Autodesk Inventor part; units mm, degrees
ref_plane "YZ Plane" through (0, 0, 0) normal (1, 0, 0) x (0, 1, 0)
ref_plane "XZ Plane" through (0, 0, 0) normal (0, 1, 0) x (-1, 0, 0)
ref_plane "XY Plane" through (0, 0, 0) normal (0, 0, 1) x (1, 0, 0)
sketch "Boceto2" plane through (0, 0, 0) normal (0, 1, 0) x (-1, 0, 0)
  line L0 (0, 0) -> (-78, 0)
  line L1 (-78, 0) -> (-78, -30)
  line L2 (-78, -30) -> (-38, -30)
  line L3 (-38, -30) -> (-38, -36)
  line L4 (-38, -36) -> (0, -36)
  line L5 (0, -36) -> (0, 0)
  dimension "d2" = 78
  dimension "d3" = 36
  dimension "d4" = 30
  dimension "d5" = 38
extrude "Extrusión1" add sketch "Boceto2" along normal blind 38
sketch "Boceto3" plane through (0, 0, -36) normal (-1, 0, 0) x (0, 0, 1)
  line L0 (0, 0) -> (36, 0) construction
  line L1 (36, 0) -> (36, 6) construction
  line L2 (36, 0) -> (36, 38) construction
  line L3 (36, 6) -> (36, 27) construction
  line L4 (36, 27) -> (36, 38) construction
  line L5 (36, 6) -> (18, 6)
  line L6 (18, 6) -> (18, 27)
  line L7 (18, 27) -> (36, 27)
  line L8 (36, 6) -> (36, 27)
  dimension "d8" = 6
  dimension "d9" = 21
  dimension "d10" = 38
  dimension "d11" = 18
extrude "Extrusión2" cut sketch "Boceto3" against normal through all
sketch "Boceto4" plane through (38, 0, -36) normal (0, 0, -1) x (-1, 0, 0)
  line L0 (38, 27) -> (38, 38) construction
  line L1 (38, 38) -> (38, 19) construction
  line L2 (38, 19) -> (19, 19) construction
  line L3 (0, 0) -> (0, 38) construction
  circle A0 centre (19, 19) radius 8
  point P0 (38, 0)
  dimension "d14" = 19
  dimension "d15" = 19
  dimension "d16" = 16
extrude "Extrusión3" cut sketch "Boceto4" against normal through all
chamfer "Chaflán1" distance 2 angle 45 4 edges at (19, 38, -36) (0, 19, -36) (19, 0, -36) (38, 19, -36)
properties part number "Practica 6"
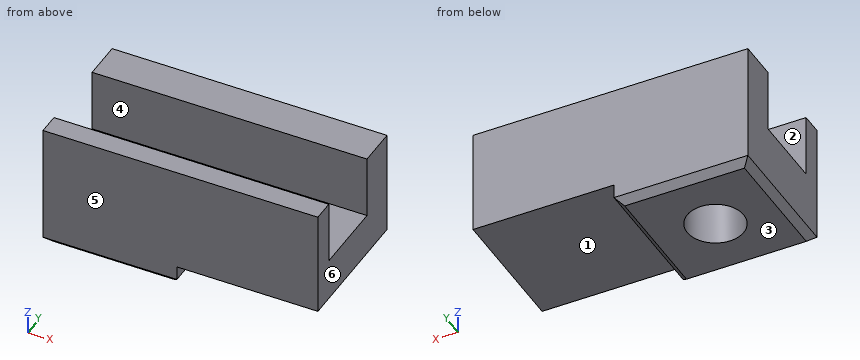
Geometry: final body of the model. Coordinates: model frame, mm. Face numbers are marked on the shaded views. A direction names the side the tool comes from. Give positions to 0.01 mm unless a question says otherwise; leave off trailing zeros. Write each loop counter-clockwise with the first axis right and the second up, starting at its lowest first coordinate (ties: lowest second). Pieces come first, ordered by that corner, then holes.
(1) Cut plane C-C, the plane x = 16.5. Return loops of the section in (y, z), then the cut area to 3 significant figures.
(2) Cut plane D-D, the plane x = 8. Return loops of the section in (y, z).
(3) First-contact query: P1, Ø6.5, axis at x = 41, y = 18, coming from the +Z side. Flat tip, straight axial feed; report the tip coordinate or a pass-through.
(4) Mould query, pull axis Y, two halves, no side actions, for the marked faces 4, 5 and 6. Classes: released by +Y, released by -Y, zero draft, split by the parting line, or undercut.
(5) Access query for the marked faces 1, 2 and 3. Directions: +Z, -Z, +X, -X, +Y, -Y. A direction counts if a zero-diameter tool reaches every point of the face in a straight line with its end or side. Return the directions, or none.
(6) Cut plane B-B, the plane z = -10.5. Return loops of the section in (x, y).
(7) Cut plane A-A, the plane y = 19. Return loops of the section in (x, z).
(8) Ray query, line 1 (Y direction, x = 19, z = -25); line 2 (X direction, y = 19, z = -21); line 3 (Y direction, x = 53, z = -10.5). Return the intervals inside material, ascending.
Values follow:
1. outline: (0, -34) - (2, -36) - (11.4, -36) - (11.4, -18) - (6, -18) - (6, 0) - (0, 0) - close; (26.6, -36) - (36, -36) - (38, -34) - (38, 0) - (27, 0) - (27, -18) - (26.6, -18) - close
1. area: 712 mm2
2. outline: (0, -34) - (2, -36) - (36, -36) - (38, -34) - (38, 0) - (27, 0) - (27, -18) - (6, -18) - (6, 0) - (0, 0) - close
3. P1: stops at z = -18
4. face 4: undercut
4. face 5: released by -Y
4. face 6: zero draft
5. face 1: -Z, +X, +Y, -Y
5. face 2: +Z, +X, -X
5. face 3: -Z, +X, -X, +Y, -Y
6. outline: (0, 0) - (78, 0) - (78, 6) - (0, 6) - close; (0, 27) - (78, 27) - (78, 38) - (0, 38) - close
7. outline: (0, -34) - (2, -36) - (11, -36) - (11, -18) - (0, -18) - close; (27, -36) - (36, -36) - (38, -34) - (38, -30) - (78, -30) - (78, -18) - (27, -18) - close
8. line 1: y = 0 to 11, 27 to 38
8. line 2: x = 0 to 11, 27 to 78
8. line 3: y = 0 to 6, 27 to 38
